from build123d import *

# Parameters (mm, degrees)
F0_R      = 5
F1_DEPTH  = 9.3
F1_TAPER  = -0.25
F3_DEPTH  = 9.3
F3_TAPER  = 1
F4_R      = 0.75
F6_W      = 4.5
F6_H      = 3
F7_DEPTH  = 7.2
F8_R      = 5.0405791626
F9_DEPTH  = 2
F10_W     = 10.0811583253
F10_H     = 12
F11_DEPTH = 1
F12_R     = 3.5


with BuildPart() as f1:
    # F0 (on Top) → F1 (new body)
    with BuildSketch(Plane.XY):
        Circle(F0_R)
        Polygon((1.7897858345, 3.1), (3.579571669, 0), (1.7897858345, -3.1), (-1.7897858345, -3.1), (-3.579571669, 0), (-1.7897858345, 3.1), align=None, mode=Mode.SUBTRACT)
        Polygon((1.7897858345, -3.1), (3.579571669, 0), (1.7897858345, 3.1), (-1.7897858345, 3.1), (-3.579571669, 0), (-1.7897858345, -3.1), align=None)
    extrude(amount=F1_DEPTH, taper=F1_TAPER)

    # F2 (on Top) → F3 (cut)
    with BuildSketch(Plane.XY):
        Polygon((1.7897858345, -3.1), (3.579571669, 0), (1.7897858345, 3.1), (-1.7897858345, 3.1), (-3.579571669, 0), (-1.7897858345, -3.1), align=None)
    extrude(amount=F3_DEPTH, taper=F3_TAPER, mode=Mode.SUBTRACT)

    # F4 (on Right) → F5 (revolve, cut)
    with BuildSketch(Plane.YZ):
        with Locations((-2.5457434822, 5.35)):
            Circle(F4_R)
    revolve(axis=Axis((0, 0, 4.7348800581), (0, 0, -1)), mode=Mode.SUBTRACT)

    # F6 (on Right) → F7 (cut, symmetric)
    with BuildSketch(Plane.YZ):
        with Locations((0, 7.8)):
            Rectangle(F6_W, F6_H)
    extrude(amount=F7_DEPTH, both=True, mode=Mode.SUBTRACT)

    # F8 (on face) → F9 (join)
    with BuildSketch(Plane.XY.offset(9.3)):
        Circle(F8_R)
    extrude(amount=F9_DEPTH)

    # F10 (on Right) → F11 (join, symmetric)
    with BuildSketch(Plane.YZ):
        with Locations((0, 17.3)):
            Rectangle(F10_W, F10_H)
    extrude(amount=F11_DEPTH, both=True)

    # F12
    f12_edges = [f1.edges().sort_by_distance(p)[0] for p in [
        (0, -5.040579, 23.3),
        (0, 5.040579, 23.3),
    ]]
    fillet(f12_edges, radius=F12_R)


solid = f1.part
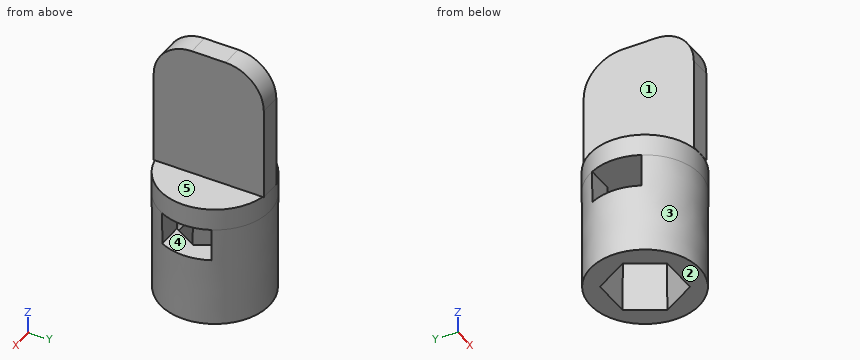
Work out the finished part from the listing and answer in its coordinate system (mm). Face numbers are marked on the shaded views. A direction names the side the tool comes from. Give positions to 0.01 mm unless a question says otherwise; leave off trailing zeros. Order: outer loops, then holes, each group sorted by start corner. A loop starts at its lowest first (then second) coordinate and runs counter-clockwise, first axis right, second up. Notation, with made-up numbers: (-21.5, 79) -> (-14.5, 79) arc R27 cw to (-14.5, 108) -> close; hole circle Ø6 at (8, 55). An arc over 180 degrees is marked (long way). Answer as a JSON object with one key per item and string values. Group by question number.
1. A tool of negligible diameter and unlimited length cuts with its end or side. For the marked faces 1, 2, 3, 4 and 5, from which of +Z, -Z, +X, -X, +Y, -Y can it reach the whole face along a straight path? Write none if from no direction.
2. Flat-ended cylindrical pins translate along their axes: pin 1 Ø1.4 at (x, y) = (-3.5, -1) entering from +Z; pin 2 Ø2.5 at (x, z) = (4, 7) entering from +Y; pin 3 Ø4 at (y, z) = (3.5, 20.5) entering from -X; pin 4 Ø2 at (x, y) = (-1.5, 2.5) entering from +Z. Find the tip coordinate at first contact, or state that the pin passes through.
3. Consider line 1 along Z through (x, y) = (4.5, -0.5); line 2 along X through (y, z) = (-1.5, 16.25); line 3 along Z through (x, y) = (1.5, 1.25). Determine where each line is inside the solid, lowest interval first. Write a range as [from, to].
4. Section A-A on z = 7.5 is taken. Determine the outline of the cut face in (x, y).
5. Section D-D on z = 19.5 is taken. Determine the outline of the cut face in (x, y), plus the area to 3 significant figures.
6. Section C-C on y = 2 is taken. Count the separate pieces of the cut face and the enclosed holes in it, plus the area to 3 significant figures.
7. Section B-B on z = 2.25 is taken. Determine the outline of the cut face in (x, y), plus the area to 3 significant figures.
Result sheet:
{
 "1": {"face 1": "+Z, -X, +Y, -Y", "face 2": "-Z, +X, -X, +Y, -Y", "face 3": "-Z", "face 4": "+X, -X", "face 5": "+Z, +X, +Y, -Y"},
 "2": {"pin 1": "stops at z = 11.3", "pin 2": "stops at y = 4.21", "pin 3": "stops at x = -1", "pin 4": "stops at z = 23.3"},
 "3": {"line 1": "z = [0, 6.3], [9.3, 11.3]", "line 2": "x = [-1, 1]", "line 3": "z = [9.3, 11.3]"},
 "4": {"outline": "(-4.5, -2.25) arc R5.03 ccw to (4.5, -2.25) -> (2.13, -2.25) -> (1.71, -2.97) -> (-1.71, -2.97) -> (-2.13, -2.25) -> close; (-4.5, 2.25) -> (-2.13, 2.25) -> (-1.71, 2.97) -> (1.71, 2.97) -> (2.13, 2.25) -> (4.5, 2.25) arc R5.03 ccw to start"},
 "5": {"outline": "(-1, -5.04) -> (1, -5.04) -> (1, 5.04) -> (-1, 5.04) -> close", "area": "20.2 mm^2"},
 "6": {"separate pieces": "3", "enclosed holes": "0", "area": "70.2 mm^2"},
 "7": {"outline": "circle Ø10.02 at (0, 0); hole (-3.53, 0) -> (-1.77, -3.06) -> (1.77, -3.06) -> (3.53, 0) -> (1.77, 3.06) -> (-1.77, 3.06) -> close", "area": "46.4 mm^2"}
}
